Work out the finished part from the listing and answer in its coordinate system (mm). Coordinates: 2 decimals unless noted, no trailing zeros. Write each loop counter-clockwise with the first axis right and the second up, starting at its lowest first coordinate (ties: lowest second). Pieces come first, ordered by that corner, then holes. Notation, with made-up numbers: M 79,-12 L 97,-12 A31 ccw 97,26 Z; hole C 4.25,-4 d1. An arc over 180 degrees is marked long. Use CSV: the item, a comma, the result in double quotes.
from build123d import *

# Parameters (mm, degrees)
F1_DEPTH = 1.5
F2_R     = 9.2
F3_R     = 85
F4_DEPTH = 0.01
F5_R     = 1.6
F6_DEPTH = 1.5


with BuildPart() as f1:
    # F0 (on Top) → F1 (new body)
    with BuildSketch(Plane.XY):
        Polygon((51.961524, 90), (-51.961524, 90), (-103.923048, 0), (-51.961524, -90), (51.961524, -90), (103.923048, 0), align=None)
    extrude(amount=F1_DEPTH)

    # F2
    f2_edges = [f1.edges().sort_by_distance(p)[0] for p in [
        (-103.923048, 0, 0.75),
        (-51.961524, 90, 0.75),
        (51.961524, 90, 0.75),
        (103.923048, 0, 0.75),
        (51.961524, -90, 0.75),
        (-51.961524, -90, 0.75),
    ]]
    fillet(f2_edges, radius=F2_R)

    # F3 (on face) → F4 (join)
    with BuildSketch(Plane.XY.offset(1.5)):
        Circle(F3_R)
    extrude(amount=F4_DEPTH)

    # F5 (on face) → F6 (cut, through all)
    with BuildSketch(Plane.XY.offset(1.5)):
        with Locations((96, 0)):
            Circle(F5_R)
        with Locations((48, 83.138439)):
            Circle(F5_R)
        with Locations((-48, 83.138439)):
            Circle(F5_R)
        with Locations((-96, 0)):
            Circle(F5_R)
        with Locations((-48, -83.138439)):
            Circle(F5_R)
        with Locations((48, -83.138439)):
            Circle(F5_R)
    extrude(amount=-F6_DEPTH, mode=Mode.SUBTRACT)


solid = f1.part
Item 1: The part is cut by section B-B (z = 1.25). Write down the section's boundary in (x, y).
Answer:
outline,"M -101.27,-4.6 L -54.62,-85.4 A9.2 ccw -46.65,-90 L 46.65,-90 A9.2 ccw 54.62,-85.4 L 101.27,-4.6 A9.2 ccw 101.27,4.6 L 54.62,85.4 A9.2 ccw 46.65,90 L -46.65,90 A9.2 ccw -54.62,85.4 L -101.27,4.6 A9.2 ccw Z; hole C -96,0 d3.2; hole C -48,-83.14 d3.2; hole C -48,83.14 d3.2; hole C 48,-83.14 d3.2; hole C 48,83.14 d3.2; hole C 96,0 d3.2"
Item 2: Given pin 1 (2.5 mm diameter, centred on x = 48, y = 83.14, fed in from +Z); pin 2 (4 mm diameter, centred on x = -48, y = 83.14, fed in from +Z), each flat-ended and moving along its own axis, determine where each tip first touches the part or whether it passes through.
Answer:
pin 1,"passes through"
pin 2,"stops at z = 1.5"
Item 3: Consider probe 1 along Y at (x, z) = (48, 0.75); probe 2 along X at (y, z) = (82.5, 1.2); probe 3 along Z at (x, y) = (54.5, -69.5). Determine where each line is inside the solid, lowest interval first.
Answer:
probe 1,"y = -89.9 to -84.74, -81.54 to 81.54, 84.74 to 89.9"
probe 2,"x = -56.29 to -49.47, -46.53 to 46.53, 49.47 to 56.29"
probe 3,"z = 0 to 1.5"
